For this review, take the finished solid that the model builds, in its own axes (mm). A direction names the side the tool comes from. Round coordinates to 2 decimals unless told otherwise and drop trailing zeros. One line per item, written item: value. Start each with the question number.
Q1. Tool access review of faces 4 (the face through (-6.925, -12.776, 0.19)), 5 (the face through (-22.58, -12.52, 3.71)), 6 (the face through (-23.669, -2.864, 1.735)): name each direction out of +Z, -Z, +X, -X, +Y, -Y from which nothing blocks a thin tool from reaching the whole face with its end or side.
Q2. For probe 1 along X at (y, z) = (-16.25, 0); probe 2 along X at (y, z) = (-9.25, 0); probe 3 along Z at (x, y) = (15, -23.5), list the stretches that pass through material, from the lowest coordinate up.
Q3. Clearance check with flat-ended pins moving along their axes: pin 1 Ø4 at (y, z) = (-7, -8.5) entering from -X; pin 2 Ø3 at (y, z) = (-19.5, -3.5) entering from +X; pin 3 Ø8 at (x, y) = (1, -10.5) entering from +Z; pin 4 Ø4 at (x, y) = (12, -13.5) entering from +Z. State where each tip first meets the part, or that it passes through.
Q4. Mouldability with a two-part tool opening along Z and no side actions: class faces 1 (the face through (-5.899, -12.522, 0.767)), 2 (the face through (-4, 0, -3)), 3 (the face through (14.944, -12.522, -9.224)) as +Z half, -Z half, draft (parallel to the pull), parting line (faces both ways), or undercut.
```python
from build123d import *

# Parameters (mm, degrees)
F1_DEPTH      = 25.4
F2_R          = 7.9375
F3_DEPTH      = 25.4
F3_TAPER      = 5
F3_DEPTH_BACK = 25.4
F4_R          = 9.525


with BuildPart() as f1:
    # F0 (on Front) → F1 (new body)
    with BuildSketch(Plane.XZ):
        with BuildLine():
            ThreePointArc((15.9420039577, -5.3261326592), (14.9211079736, -9.2769096997), (12.7, -12.7))
            ThreePointArc((12.7, -12.7), (12.5948783029, -14.7822408301), (14.6158441263, -15.2945635671))
            ThreePointArc((14.6158441263, -15.2945635671), (17.697106564, -10.8437100374), (19.1037159776, -5.6163086455))
            ThreePointArc((19.1037159776, -5.6163086455), (10.77478978, 7.4777303194), (-3.9952923544, 2.7164760977))
            ThreePointArc((-3.9952923544, 2.7164760977), (-5.934088224, 0.7499909222), (-8.6788133112, 0.4458896807))
            Line((-8.6788133112, 0.4458896807), (-25.5047661099, 4.3984803395))
            Line((-25.5047661099, 4.3984803395), (-26.9643777894, 0.8821428277))
            Line((-26.9643777894, 0.8821428277), (-9.3699563909, -6.421201314))
            ThreePointArc((-9.3699563909, -6.421201314), (-6.8229957257, -8.720792311), (-6.2949665087, -12.1114135711))
            ThreePointArc((-6.2949665087, -12.1114135711), (-2.3576029431, -15.767977681), (-0.7614577713, -10.6371284795))
            ThreePointArc((-0.7614577713, -10.6371284795), (3.5871947735, 4.6083370701), (15.9420039577, -5.3261326592))
        make_face()
    extrude(amount=F1_DEPTH)

    # F2 (on face) → F3 (cut, two sides)
    with BuildSketch(Plane(origin=(-0.354609422, 0, -1.5095520662), x_dir=(0.9735003954, 0, -0.22868533), z_dir=(0.22868533, 0, 0.9735003954))) as f3_sk:
        with Locations((-14.7222678204, -12.7)):
            Circle(F2_R)
    extrude(amount=-F3_DEPTH, taper=F3_TAPER, mode=Mode.SUBTRACT)
    extrude(f3_sk.sketch, amount=F3_DEPTH_BACK, mode=Mode.SUBTRACT)

    # F4
    f4_edges = [f1.edges().sort_by_distance(p)[0] for p in [
        (-26.234572, 0, 2.640312),
        (-26.234572, -25.4, 2.640312),
    ]]
    fillet(f4_edges, radius=F4_R)


solid = f1.part
```
Result set:
1. face 4: +Z
1. face 5: +Z, +Y, -Y
1. face 6: +Z, -X, +Y
2. probe 1: x = -24.84 to -22.06, -7.86 to -1.93, 14.87 to 18.35
2. probe 2: x = -24.84 to -22.11, -7.8 to -1.93, 14.87 to 18.35
2. probe 3: z = -14.89 to -9.09, -0.25 to 4.93
3. pin 1: stops at x = -9.19
3. pin 2: stops at x = 19.16
3. pin 3: stops at z = 8.15
3. pin 4: stops at z = 7.73
4. face 1: +Z half
4. face 2: draft
4. face 3: undercut
